```python
from build123d import *

# Parameters (mm, degrees)
SKETCH1_W           = 26
SKETCH1_H           = 2.5
BOSS_EXTRUDE1_DEPTH = 8.5
SKETCH2_W           = 1
SKETCH2_H           = 1
CUT_EXTRUDE1_DEPTH  = 5
CHAMFER1_SIZE       = 0.5
SKETCH3_R           = 0.25
BOSS_EXTRUDE2_DEPTH = 6.5


with BuildPart() as part:
    # Sketch1 → Boss-Extrude1 (new body)
    with BuildSketch(Plane(origin=(0, 0, 0), x_dir=(1, 0, 0), z_dir=(0, 1, 0))):
        with Locations((13, 1.25)):
            Rectangle(SKETCH1_W, SKETCH1_H)
    extrude(amount=BOSS_EXTRUDE1_DEPTH)

    # Sketch2 → Cut-Extrude1 (cut)
    with BuildSketch(Plane(origin=(0, 8.5, 0), x_dir=(1, 0, 0), z_dir=(0, 1, 0))):
        with Locations((1.9545, 1.25)):
            Rectangle(SKETCH2_W, SKETCH2_H)
        with Locations((4.409, 1.25)):
            Rectangle(SKETCH2_W, SKETCH2_H)
        with Locations((6.8635, 1.25)):
            Rectangle(SKETCH2_W, SKETCH2_H)
        with Locations((9.318, 1.25)):
            Rectangle(SKETCH2_W, SKETCH2_H)
        with Locations((11.7725, 1.25)):
            Rectangle(SKETCH2_W, SKETCH2_H)
        with Locations((14.227, 1.25)):
            Rectangle(SKETCH2_W, SKETCH2_H)
        with Locations((16.6815, 1.25)):
            Rectangle(SKETCH2_W, SKETCH2_H)
        with Locations((19.136, 1.25)):
            Rectangle(SKETCH2_W, SKETCH2_H)
        with Locations((21.5905, 1.25)):
            Rectangle(SKETCH2_W, SKETCH2_H)
        with Locations((24.045, 1.25)):
            Rectangle(SKETCH2_W, SKETCH2_H)
    extrude(amount=-CUT_EXTRUDE1_DEPTH, mode=Mode.SUBTRACT)

    # Chamfer1
    chamfer1_edges = [part.edges().sort_by_distance(p)[0] for p in [
        (21.0905, 8.5, -1.25),
        (21.5905, 8.5, -0.75),
        (22.0905, 8.5, -1.25),
        (21.5905, 8.5, -1.75),
        (23.545, 8.5, -1.25),
        (24.045, 8.5, -0.75),
        (24.545, 8.5, -1.25),
        (24.045, 8.5, -1.75),
        (1.4545, 8.5, -1.25),
        (1.9545, 8.5, -0.75),
        (2.4545, 8.5, -1.25),
        (1.9545, 8.5, -1.75),
        (3.909, 8.5, -1.25),
        (4.409, 8.5, -0.75),
        (4.909, 8.5, -1.25),
        (4.409, 8.5, -1.75),
        (6.3635, 8.5, -1.25),
        (6.8635, 8.5, -0.75),
        (7.3635, 8.5, -1.25),
        (6.8635, 8.5, -1.75),
        (8.818, 8.5, -1.25),
        (9.318, 8.5, -0.75),
        (9.818, 8.5, -1.25),
        (9.318, 8.5, -1.75),
        (11.2725, 8.5, -1.25),
        (11.7725, 8.5, -0.75),
        (12.2725, 8.5, -1.25),
        (11.7725, 8.5, -1.75),
        (13.727, 8.5, -1.25),
        (14.227, 8.5, -0.75),
        (14.727, 8.5, -1.25),
        (14.227, 8.5, -1.75),
        (16.1815, 8.5, -1.25),
        (16.6815, 8.5, -0.75),
        (17.1815, 8.5, -1.25),
        (16.6815, 8.5, -1.75),
        (18.636, 8.5, -1.25),
        (19.136, 8.5, -0.75),
        (19.636, 8.5, -1.25),
        (19.136, 8.5, -1.75),
    ]]
    chamfer(chamfer1_edges, length=CHAMFER1_SIZE)

    # Sketch3 → Boss-Extrude2 (add)
    with BuildSketch(Plane(origin=(0, 3.5, 0), x_dir=(1, 0, 0), z_dir=(0, 1, 0))):
        with Locations((1.9545, 1.25)):
            Circle(SKETCH3_R)
        with Locations((4.409, 1.25)):
            Circle(SKETCH3_R)
        with Locations((6.8635, 1.25)):
            Circle(SKETCH3_R)
        with Locations((9.183250215, 1.115250215)):
            Circle(SKETCH3_R)
        with Locations((11.7725, 1.25)):
            Circle(SKETCH3_R)
        with Locations((14.227, 1.25)):
            Circle(SKETCH3_R)
        with Locations((16.6815, 1.25)):
            Circle(SKETCH3_R)
        with Locations((19.136, 1.25)):
            Circle(SKETCH3_R)
        with Locations((21.5905, 1.25)):
            Circle(SKETCH3_R)
        with Locations((24.045, 1.25)):
            Circle(SKETCH3_R)
    extrude(amount=-BOSS_EXTRUDE2_DEPTH)


solid = part.part
```
Geometry check sheet. Reference: the model listing, model coordinates, mm. A direction names the side the tool comes from. Give positions to 0.01 mm unless a question says otherwise; leave off trailing zeros. Write item = value, one per line. Start each with the question number.
1) Access from +Z, -Z, +X, -X, +Y, -Y to the whole of each face (thin tool, end or side, straight path). Record for faces 3 (the flat face through (19, 3.5, -1)), 4 (the flat face through (13, 4, 0)).
2) Draft check along X on faces 1 (the flat face through (12, 3.5, -1)), 2 (the flat face through (13, 4, -2.5)). Enter one of: released by +X, released by -X, zero draft, split by the parting line, or undercut.
3) Gauge pin test, flat ends, axial feed: pin 1 Ø0.8 at (x, z) = (7, -1.5) entering from +Y; pin 2 Ø0.8 at (x, z) = (11.5, -1) entering from +Y; pin 3 Ø1.1 at (x, z) = (16.5, -1) entering from +Y. Record the tip position at first contact, or that the pin passes through.
4) Section check A-A (y = -1.5). Count the separate pieces of the cut face and the enclosed holes in it, then the cut area to 3 significant figures.
5) Scan lines: L1, parallel to Y at x = 9, z = -1.1; L2, parallel to Y at x = 3.25, z = -2.2; L3, parallel to Z at x = 21.75, y = -1. Record each from-to range of solid material in increasing order.
Geometry check:
q1.face_3 = +Y
q1.face_4 = +Z, +X, -X, +Y, -Y
q2.face_1 = undercut
q2.face_2 = zero draft
q3.pin_1 = 8.15
q3.pin_2 = 8.17
q3.pin_3 = 8.3
q4.separate_pieces = 10
q4.enclosed_holes = 0
q4.area = 1.96 mm2
q5.L1 = -3 to 3.5
q5.L2 = 0 to 8.5
q5.L3 = -1.44 to -1.06
